Could you check a few things on this model? Use its own coordinates, in mm. Face numbers are marked on the shaded views. A direction names the side the tool comes from. Coordinates: 2 decimals unless noted, no trailing zeros. Write each loop counter-clockwise with the first axis right and the second up, starting at its lowest first coordinate (ties: lowest second). Pieces come first, ordered by that corner, then holes.
Autodesk Fusion 360 part; units mm, degrees
sketch "Sketch1" plane through (0, 0, 0) normal (0, 1, 0) x (1, 0, 0)
  circle A0 centre (0, 0) radius 7.2
  circle A1 centre (0, 0) radius 2.55
  line L0 (7.2, 0) -> (2.55, 0)
  line L1 (2.55, 0) -> (2.55, -28.2)
  line L2 (2.55, -28.2) -> (7.2, -28.2)
  line L3 (7.2, -28.2) -> (7.2, 0)
  line L4 (7.2, -28.2) -> (-3.3, -28.2)
  line L5 (-3.3, -28.2) -> (-3.3, -23.55)
  line L6 (-3.3, -23.55) -> (7.2, -23.55)
  line L7 (7.2, -23.55) -> (7.2, -28.2)
  line L8 (2.55, 0) -> (-7.2, 0)
  line L9 (7.2, -5.8) -> (7.2, -1.15)
  line L10 (7.2, -13.9742) -> (42.0463, -10.6976)
  line L11 (42.0463, -10.6976) -> (41.6194, -6.1577)
  line L12 (41.6194, -6.1577) -> (6.7731, -9.4343)
  line L13 (6.7731, -9.4343) -> (7.2, -13.9742)
  line L14 (42.0463, -10.6976) -> (37.8278, -8.7415)
  line L15 (37.8278, -8.7415) -> (40.0153, -4.024)
  line L16 (40.0153, -4.024) -> (44.2339, -5.9802)
  line L17 (44.2339, -5.9802) -> (42.0463, -10.6976)
  dimension "d1" = 14.4
  dimension "d2" = 5.1
  dimension "d3" = 4.65
  dimension "d4" = 28.2
  dimension "d5" = 10.5
  dimension "d6" = 4.65
  dimension "d16" = 35
  dimension "d17" = 4.56
  dimension "d18" = 4.65
  dimension "d19" = 5.2
extrude "Extrude1" add sketch "Sketch1" along normal blind 4.65 contours A0 A1 L0 L8 | A0 L1 L3 L6 L9 L12 L13 | A0 L0 L1 | L1 L2 L3 L4 L6 L7 | L1 L4 L5 L6 | L3 L10 L12 L14 L15 | L3 L12 L13 | L11 L12 L15 L16 L17 | L11 L12 L14 L15
fillet "Fillet1" radius 2 3 edges at (40.0153, 2.325, 4.024) (44.2339, 2.325, 5.9802) (42.0463, 2.325, 10.6976)
fillet "Fillet2" radius 2 1 edges at (7.2, 2.325, 28.2)
fillet "Fillet3" radius 2 2 edges at (-0.375, 4.65, 23.55) (-0.375, 0, 23.55)
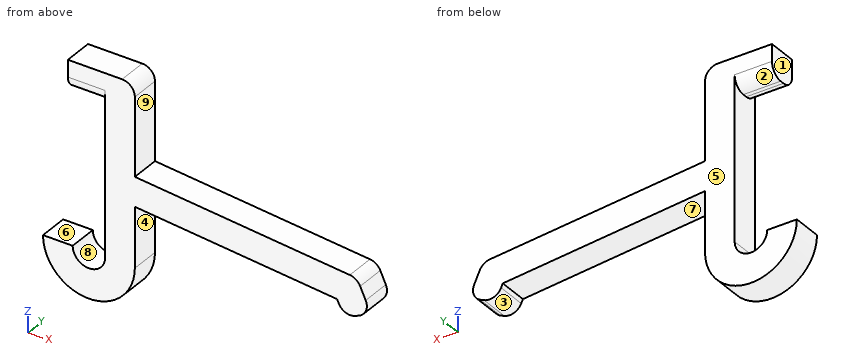
Item 1: I want a section at B-B, the plane z = 18. List the corners of the cut face in (x, y) for me, then the cut area to 3 significant figures.
Item 2: Which directions (+Z, -Z, +X, -X, +Y, -Y) give clear straight access to the entire face, cutting with the end or side of a thin tool? Please do the marked faces 5, 6, 7, 8 and 9.
Item 3: If we mould it in two halves opening along X, with no side actions, what happens to the marked faces 1, 2, 3 and 4? For each: released by +X, released by -X, zero draft, split by the parting line, or undercut.
Item 4: Will these pins go through, and if not, where does the flat tip stop? pin 1 Ø2.5 at (y, z) = (2.5, 21.5) entering from +X; pin 2 Ø1.4 at (y, z) = (2, 18) entering from -X; pin 3 Ø2 at (x, y) = (30, 1.5) entering from -Z.
Item 5: I want a section at A-A, the plane x = 0. List the corners of the cut face in (y, z) for me, then the cut area to 3 significant figures.
Item 6: If I drill on line 1 along X through (y, z) = (4.35, 17); line 2 along X through (y, z) = (2.7, -0.5); line 3 along Z through (x, y) = (30.5, 3.2), over which ranges is the centre line in solid material (lowest first)?
Item 7: I want a section at C-C, the plane x = 37. List the corners of the cut face in (y, z) for me, then the cut area to 3 significant figures.
Taken from the geometry:
1. outline: (2.55, 0) - (7.2, 0) - (7.2, 4.65) - (2.55, 4.65) - close
1. area: 21.6 mm2
2. face 5: +Z, -Z, +X, -X, +Y
2. face 6: -X, +Y, -Y
2. face 7: -Z, +Y, -Y
2. face 8: +Y, -Y
2. face 9: +Z, +X, +Y, -Y
3. face 1: released by -X
3. face 2: zero draft
3. face 3: undercut
3. face 4: undercut
4. pin 1: stops at x = 7.2
4. pin 2: stops at x = 2.55
4. pin 3: stops at z = 7.16
5. outline: (0, -7.2) - (4.65, -7.2) - (4.65, -2.55) - (0, -2.55) - close; (0, 25.55) arc R2 ccw to (2, 23.55) - (2.65, 23.55) arc R2 ccw to (4.65, 25.55) - (4.65, 28.2) - (0, 28.2) - close
5. area: 41.5 mm2
6. line 1: x = 2.55 to 7.2
6. line 2: x = -7.18 to -2.5, 2.5 to 7.18
6. line 3: z = 7.2 to 11.78
7. outline: (0, 6.59) - (4.65, 6.59) - (4.65, 11.17) - (0, 11.17) - close
7. area: 21.3 mm2
